```python
from build123d import *

# Parameters (mm, degrees)
PAD_DEPTH       = 24
FILLET_R        = 3
SKETCH001_R     = 8.25
SKETCH001_R_2   = 1.1
POCKET_DEPTH    = 5
SKETCH002_R     = 1.05
SKETCH002_R_2   = 2
POCKET001_DEPTH = 5


with BuildPart() as part:
    # Sketch → Pad (new body, symmetric)
    with BuildSketch(Plane.XY):
        Polygon((-3, 31), (0, 31), (0, 0), (-18, 0), (-18, 3), (-3, 3), align=None)
    extrude(amount=PAD_DEPTH, both=True)

    # Fillet
    fillet_edges = [part.edges().sort_by_distance(p)[0] for p in [
        (-1.5, 31, 24),
        (-1.5, 31, -24),
        (-18, 1.5, -24),
        (-18, 1.5, 24),
    ]]
    fillet(fillet_edges, radius=FILLET_R)

    # Sketch001 (on Face5 of Fillet) → Pocket (cut)
    with BuildSketch(Plane.YZ):
        with Locations((18, 13.5)):
            Circle(SKETCH001_R)
        with Locations((18, -13.5)):
            Circle(SKETCH001_R)
        with Locations((9.5, 20.5)):
            Circle(SKETCH001_R_2)
        with Locations((26.5, -20.5)):
            Circle(SKETCH001_R_2)
    extrude(amount=-POCKET_DEPTH, mode=Mode.SUBTRACT)

    # Sketch002 (on Face8 of Pocket) → Pocket001 (cut)
    with BuildSketch(Plane(origin=(0, 3, 0), x_dir=(-1, 0, 0), z_dir=(0, 1, 0))):
        with Locations((12, 11)):
            Circle(SKETCH002_R)
        with Locations((12, -11)):
            Circle(SKETCH002_R)
        with Locations((12, 0)):
            Circle(SKETCH002_R_2)
    extrude(amount=-POCKET001_DEPTH, mode=Mode.SUBTRACT)


solid = part.part
```
Design review of the part built by this model. Coordinates are the model's own, in mm. A direction names the side the tool comes from. Coordinates: 2 decimals unless noted, no trailing zeros. Loops run counter-clockwise (first coordinate to the right, second up) from the corner with the lowest first, then second, coordinate; pieces in that order, holes last. Notation, with made-up numbers: M 48.5,-2.75 L 59.5,-2.75 A13 cw 59.5,5.25 Z; hole C 44.5,3.5 d9. An arc over 180 degrees is marked long. One line per question, with ' | ' between items.
(1) We need section A-A (z = 13.5). Give the boundary of the cut face in (x, y), and give its area (3 significant figures).
Filled in:
outline: M -18,0 L 0,0 L 0,9.75 L -3,9.75 L -3,3 L -18,3 Z; M -3,26.25 L 0,26.25 L 0,31 L -3,31 Z | area: 88.5 mm^2
(2) For pin 1 Ø5 at (x, z) = (-6, -9) entering from -Y; pin 2 Ø14 at (y, z) = (15.5, 9.5) entering from -X; pin 3 Ø4.5 at (x, z) = (-12, 0) entering from +Y, all flat-tipped, find the tip position at first contact; note any pin that passes through.
Filled in:
pin 1: stops at y = 0 | pin 2: stops at x = -3 | pin 3: stops at y = 3
(3) We need section D-D (z = 20.5). Give the boundary of the cut face in (x, y).
Filled in:
outline: M -18,0 L 0,0 L 0,8.4 L -3,8.4 L -3,3 L -18,3 Z; M -3,10.6 L 0,10.6 L 0,13.63 L -3,13.63 Z; M -3,22.37 L 0,22.37 L 0,31 L -3,31 Z
(4) Wall thickness on probe 1 along Y at (x, z) = (-8, 20.5); probe 2 along Z at (x, y) = (-1.75, 20); probe 3 along X at (y, z) = (10, 4.5): over which ranges is each line inside the solid? List them lowest first.
Filled in:
probe 1: y = 0 to 3 | probe 2: z = -24 to -21.5, -5.5 to 5.5, 21.5 to 24 | probe 3: x = -3 to 0
(5) Draft analysis for pull direction Z (two halves, no side actions). For faces 3 (the face through (-17.1, 1.52, 23.14)), 4 (the face through (0, 16, 0)), 5 (the face through (-12.56, 1.52, -10.11)), state which applies: released by +Z, released by -Z, zero draft, split by the parting line, or undercut.
Filled in:
face 3: released by +Z | face 4: zero draft | face 5: undercut
(6) Machinability: for faces 1 (the face through (-3, 17, 0)), 2 (the face through (-2, 31, 0)), which of the approach directions +Z, -Z, +X, -X, +Y, -Y give a long, thin tool a straight path to every point of the face, cutting with its end or side? Answer none if there is none.
Filled in:
face 1: +Z, -Z, -X, +Y | face 2: +Z, -Z, +X, -X, +Y
(7) We need section C-C (x = -12). Give the boundary of the cut face in (y, z), and give its area (3 significant figures).
Filled in:
outline: M 0,-24 L 3,-24 L 3,-12.05 L 0,-12.05 Z; M 0,-9.95 L 3,-9.95 L 3,-2 L 0,-2 Z; M 0,2 L 3,2 L 3,9.95 L 0,9.95 Z; M 0,12.05 L 3,12.05 L 3,24 L 0,24 Z | area: 119 mm^2
(8) We need section B-B (y = 18). Give the boundary of the cut face in (x, z).
Filled in:
outline: M -3,-24 L 0,-24 L 0,-21.75 L -3,-21.75 Z; M -3,-5.25 L 0,-5.25 L 0,5.25 L -3,5.25 Z; M -3,21.75 L 0,21.75 L 0,24 L -3,24 Z
